from build123d import *

# Parameters (mm, degrees)
F0_W     = 1890
F0_H     = 180
F1_DEPTH = 220
F2_W     = 1884
F2_H     = 174
F3_DEPTH = 217
F4_R     = 15
F5_DEPTH = 3


with BuildPart() as f1:
    # F0 (on Top) → F1 (new body)
    with BuildSketch(Plane.XY):
        with Locations((898.785665, 53.946961)):
            Rectangle(F0_W, F0_H)
    extrude(amount=F1_DEPTH)

    # F2 (on face) → F3 (cut)
    with BuildSketch(Plane.XY.offset(220)):
        with Locations((898.785665, 53.946961)):
            Rectangle(F2_W, F2_H)
    extrude(amount=-F3_DEPTH, mode=Mode.SUBTRACT)

    # F4 (on face) → F5 (cut, through all)
    with BuildSketch(Plane.XZ.offset(36.053039)):
        with Locations((293.785665, 175)):
            Circle(F4_R)
        with Locations((1783.785665, 175)):
            Circle(F4_R)
    extrude(amount=-F5_DEPTH, mode=Mode.SUBTRACT)


solid = f1.part
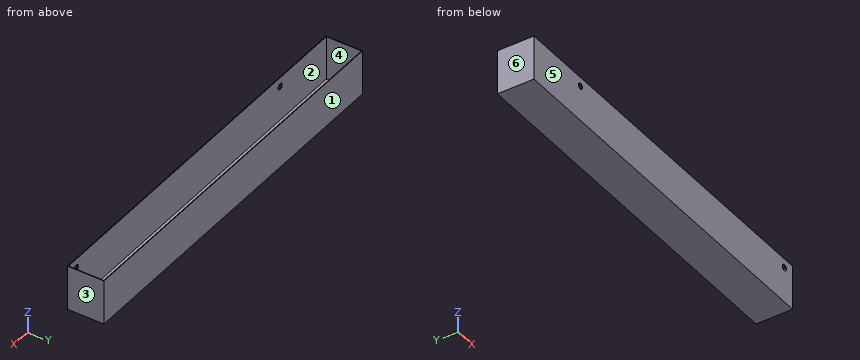
Verification items for the finished model (mm, model axes). Face numbers are marked on the shaded views. A direction names the side the tool comes from. Round coordinates to 2 decimals unless told otherwise and drop trailing zeros. Order: outer loops, then holes, each group sorted by start corner. A loop starts at its lowest first (then second) coordinate and runs counter-clockwise, first axis right, second up. Notation, with made-up numbers: (22.5, 70.5) -> (56.5, 70.5) arc R6 cw to (56.5, 77.5) -> close; hole circle Ø10 at (6.25, 62.5). An arc over 180 degrees is marked (long way). Put each result on its own line as item: value.
1) Mould release check, pull along X, two halves, no side actions. Record for the marked faces 3, 4, 5 and 6: +X half, -X half, draft (parallel to the pull), parting line (faces both ways), or undercut.
Final values:
face 3: +X half
face 4: undercut
face 5: draft
face 6: -X half
2) Material ranges on line 1 (X direction, y = -16.5, z = 55.5); line 2 (Y direction, x = 1196.5, z = 96.5); line 3 (Z direction, x = 1207, y = 91), recorded low to high.
Final values:
line 1: x = -46.21 to -43.21, 1840.79 to 1843.79
line 2: y = -36.05 to -33.05, 140.95 to 143.95
line 3: z = 0 to 3
3) Section check A-A (y = 20). Record the cut outline in (x, z), then the cut area to 3 significant figures.
Final values:
outline: (-46.21, 0) -> (1843.79, 0) -> (1843.79, 220) -> (1840.79, 220) -> (1840.79, 3) -> (-43.21, 3) -> (-43.21, 220) -> (-46.21, 220) -> close
area: 6,970 mm^2
4) Section check B-B (z = 27.5). Record the cut outline in (x, y).
Final values:
outline: (-46.21, -36.05) -> (1843.79, -36.05) -> (1843.79, 143.95) -> (-46.21, 143.95) -> close; hole (-43.21, -33.05) -> (1840.79, -33.05) -> (1840.79, 140.95) -> (-43.21, 140.95) -> close
5) Depth check by flat-ended pin: pin 1 (10 mm diameter, centred on x = 1125.5, y = 72, fed in from +Z). Enter the tip coordinate at first touch or a pass-through.
Final values:
pin 1: stops at z = 3
6) Section check C-C (x = 703). Record the cut outline in (y, z), then the cut area to 3 significant figures.
Final values:
outline: (-36.05, 0) -> (143.95, 0) -> (143.95, 220) -> (140.95, 220) -> (140.95, 3) -> (-33.05, 3) -> (-33.05, 220) -> (-36.05, 220) -> close
area: 1,840 mm^2
7) Set-up check for the marked faces 1 and 2: record each of +Z, -Z, +X, -X, +Y, -Y from which the full face is reachable in a straight line by a thin tool's end or side.
Final values:
face 1: +Z, -Z, +X, -X, +Y
face 2: +Z
